For this review, take the finished solid that the model builds, in its own axes (mm). Give positions to 0.01 mm unless a question says otherwise; leave off trailing zeros. Loops run counter-clockwise (first coordinate to the right, second up) from the corner with the lowest first, then second, coordinate; pieces in that order, holes last. Notation, with made-up numbers: (55.25, 56.25) - (109.25, 56.25) arc R5 cw to (109.25, 62.25) - close; hole circle Ø2 at (-29, 27). An arc over 180 degrees is marked (long way). Answer in a Markdown table with one row per item.
```python
from build123d import *

# Parameters (mm, degrees)
SKETCH1_W           = 29
SKETCH1_H           = 36
BOSS_EXTRUDE1_DEPTH = 4.75
SKETCH2_R           = 0.4
BOSS_EXTRUDE2_DEPTH = 4.75
FILLET1_R           = 1


with BuildPart() as part:
    # Sketch1 → Boss-Extrude1 (new body)
    with BuildSketch(Plane(origin=(0, 0, 0), x_dir=(1, 0, 0), z_dir=(0, 1, 0))):
        Rectangle(SKETCH1_W, SKETCH1_H)
    extrude(amount=BOSS_EXTRUDE1_DEPTH)

    # Sketch2 → Boss-Extrude2 (add)
    with BuildSketch(Plane(origin=(0, 0, -18), x_dir=(-1, 0, 0), z_dir=(0, 0, -1))):
        with Locations((1.5, 2.375)):
            Circle(SKETCH2_R)
        with Locations((-1.5, 2.375)):
            Circle(SKETCH2_R)
    extrude(amount=BOSS_EXTRUDE2_DEPTH)

    # Fillet1
    fillet1_edges = [part.edges().sort_by_distance(p)[0] for p in [
        (-14.5, 4.75, 0),
        (14.5, 4.75, 0),
        (-14.5, 0, 0),
        (14.5, 0, 0),
    ]]
    fillet(fillet1_edges, radius=FILLET1_R)


solid = part.part
```
1. Clearance check with a flat-ended pin moving along its axis: pin 1 (1.4 mm diameter, centred on x = -7, y = 3, fed in from -Z). State where the tip first meets the part, or that it passes through.
Values:
| item | result |
|---|---|
| pin 1 | stops at z = -18 |
2. Wall thickness on line 1 (Z direction, x = -4, y = 0.95); line 2 (X direction, y = 0.9, z = -3): over which ranges is each line inside the solid? List them lowest first. Write a range as [from, to].
Values:
| item | result |
|---|---|
| line 1 | z = [-18, 18] |
| line 2 | x = [-14.49, 14.49] |
3. We need section A-A, the plane x = 6. Give the boundary of the cut face in (y, z).
Values:
| item | result |
|---|---|
| outline | (0, -18) - (4.75, -18) - (4.75, 18) - (0, 18) - close |
4. We need section B-B, the plane y = 0.55. Give the boundary of the cut face in (x, z), and give its area (3 significant figures).
Values:
| item | result |
|---|---|
| outline | (-14.39, -18) - (14.39, -18) - (14.39, 18) - (-14.39, 18) - close |
| area | 1,040 mm^2 |
